The listing builds one solid part. Answer for the finished solid, in the listing's coordinates (mm). A direction names the side the tool comes from. Give positions to 0.01 mm unless a question says otherwise; leave off trailing zeros. Write each loop counter-clockwise with the first axis right and the second up, starting at its lowest first coordinate (ties: lowest second). Pieces come first, ordered by that corner, then holes. Notation, with made-up numbers: (-36.75, 71) - (-13.75, 71) arc R30 cw to (-13.75, 96) - close; hole circle Ø5 at (49.25, 31). An arc over 180 degrees is marked (long way). Return JSON: item names as keys, results as strings.
from build123d import *

# Parameters (mm, degrees)
F1_DEPTH = 19.05
F2_R     = 2.5
F3_DEPTH = 22
F5_DEPTH = 25
F7_DEPTH = 5
F8_R     = 1.8568549072
F9_DEPTH = 5


with BuildPart() as f1:
    # F0 (on Right) → F1 (new body)
    with BuildSketch(Plane.YZ):
        with BuildLine():
            Line((25, 0), (25, 1.9))
            Line((25, 1.9), (-25, 1.9))
            ThreePointArc((-25, 1.9), (-27.3925963531, 3.5206705817), (-26.8228433758, 6.3537734721))
            Line((-26.8228433758, 6.3537734721), (-9.338179633, 23.8384372149))
            Line((-9.338179633, 23.8384372149), (-10.6816825172, 25.1819400992))
            Line((-10.6816825172, 25.1819400992), (-28.3593520469, 7.5042705695))
            ThreePointArc((-28.3593520469, 7.5042705695), (-29.2640479302, 2.5952189514), (-25.0000004369, 0))
            Line((-25.0000004369, 0), (25, 0))
        make_face()
    extrude(amount=F1_DEPTH)

    # F2 (on face) → F3 (cut)
    with BuildSketch(Plane(origin=(0, 0, 0), x_dir=(1, 0, 0), z_dir=(0, 0, -1))):
        with BuildLine():
            Line((7.025, -5.5), (7.025, -20.5))
            ThreePointArc((7.025, -20.5), (9.525, -23), (12.025, -20.5))
            Line((12.025, -20.5), (12.025, -5.5))
            ThreePointArc((12.025, -5.5), (9.525, -3), (7.025, -5.5))
        make_face()
        with Locations((9.525, 7)):
            Circle(F2_R)
    extrude(amount=-F3_DEPTH, mode=Mode.SUBTRACT)

    # F4 (on face) → F5 (cut)
    with BuildSketch(Plane(origin=(0, 0, 0), x_dir=(1, 0, 0), z_dir=(0, 0, -1))):
        with BuildLine():
            ThreePointArc((2.0190405194, -25), (0.8550772375, -24.1079124506), (0, -22.9164958))
            Line((0, -22.9164958), (0, -25))
            Line((0, -25), (2.0190405194, -25))
        make_face()
        with BuildLine():
            ThreePointArc((19.05, -22.9164958), (18.1949227625, -24.1079124506), (17.0309594806, -25))
            Line((17.0309594806, -25), (19.05, -25))
            Line((19.05, -25), (19.05, -22.9164958))
        make_face()
    extrude(amount=-F5_DEPTH, mode=Mode.SUBTRACT)

    # F6 (on face) → F7 (cut)
    with BuildSketch(Plane(origin=(0, -17.9318113082, 17.9318113082), x_dir=(1, 0, 0), z_dir=(0, -0.7071067812, 0.7071067812))):
        with BuildLine():
            ThreePointArc((0, 7.3159923777), (0.8932364996, 9.0155780009), (2.3611190263, 10.2532304652))
            Line((2.3611190263, 10.2532304652), (0, 10.2532304652))
            Line((0, 10.2532304652), (0, 7.3159923777))
        make_face()
        with BuildLine():
            Line((19.05, 10.2532304652), (16.6888809737, 10.2532304652))
            ThreePointArc((16.6888809737, 10.2532304652), (18.1567635004, 9.0155780009), (19.05, 7.3159923777))
            Line((19.05, 7.3159923777), (19.05, 10.2532304652))
        make_face()
    extrude(amount=-F7_DEPTH, mode=Mode.SUBTRACT)

    # F8 (on face) → F9 (cut)
    with BuildSketch(Plane(origin=(0, -17.9318113082, 17.9318113082), x_dir=(1, 0, 0), z_dir=(0, -0.7071067812, 0.7071067812))):
        with Locations((4.5, 2.7532304652)):
            Circle(F8_R)
        with Locations((14.55, 2.7532304652)):
            Circle(F8_R)
    extrude(amount=-F9_DEPTH, mode=Mode.SUBTRACT)


solid = f1.part
Item 1: A cutting plane is placed at A-A on y = -7. Determine the outline of the cut face in (x, z) (3 decimals), then the cut area to 3 significant figures.
Answer below:
{"outline": "(0, 0) - (7.025, 0) - (7.025, 1.9) - (0, 1.9) - close; (12.025, 0) - (19.05, 0) - (19.05, 1.9) - (12.025, 1.9) - close", "area": "26.7 mm²"}
Item 2: Consider L1, parallel to X at y = -7, z = 0.7 (3 decimals); L2, parallel to Z at x = 13.5, y = 11; L3, parallel to Z at x = 16, y = -10. Determine where each line is inside the solid, lowest interval first.
Answer below:
{"L1": "x = 0 to 7.025, 12.025 to 19.05", "L2": "z = 0 to 1.9", "L3": "z = 0 to 1.9, 23.18 to 24.5"}
Item 3: A cutting plane is placed at D-D on y = 0. Determine the outline of the cut face in (x, z), then the cut area to 3 significant figures.
Answer below:
{"outline": "(0, 0) - (19.05, 0) - (19.05, 1.9) - (0, 1.9) - close", "area": "36.2 mm²"}
Item 4: Flat-ended cylindrical pins translate along their axes: P1, Ø6, axis at x = 16, y = -18.5, coming from the +Z side; P2, Ø5.5, axis at x = 7.5, y = -6.5, coming from the -Z side; P3, Ø2, axis at x = 6.5, z = 15, coming from the -Y side. Find the tip coordinate at first contact, or state that the pin passes through.
Answer below:
{"P1": "stops at z = 20.35", "P2": "stops at z = 0", "P3": "stops at y = -21.86"}
Item 5: A cutting plane is placed at B-B on x = 5.25. Determine the outline of the cut face in (y, z).
Answer below:
{"outline": "(-28.36, 7.5) arc R4.4 ccw to (-25, 0) - (25, 0) - (25, 1.9) - (-25, 1.9) arc R2.61 cw to (-26.82, 6.35) - (-15.84, 17.33) - (-17.19, 18.68) - close; (-14.78, 21.08) - (-13.44, 19.74) - (-9.34, 23.84) - (-10.68, 25.18) - close"}
Item 6: For faces 1 (the face through (9, 0, 1.9)), 2 (the face through (9.6, 3, 0.9)), 3 (the face through (16.32, -14.93, 19.61)), determine the directions among +Z, -Z, +X, -X, +Y, -Y from which every point of the face is accessible in a straight line to the end or side of a thin tool.
Answer below:
{"face 1": "+X, -X, +Y", "face 2": "+Z, -Z", "face 3": "none"}
Item 7: The mould has two halves that part along Z. Classify faces 4 (the face through (9.392, -19.397, 16.467)), 5 (the face through (19.05, -9, 1)), 6 (the face through (9.392, -18.203, 14.974)), 7 (the face through (9.392, -29.294, 2.663)): +Z half, -Z half, draft (parallel to the pull), parting line (faces both ways), or undercut.
Answer below:
{"face 4": "+Z half", "face 5": "draft", "face 6": "undercut", "face 7": "parting line"}
Item 8: A cutting plane is placed at C-C on y = -26. Determine the outline of the cut face in (x, z).
Answer below:
{"outline": "(0, 0.06) - (19.05, 0.06) - (19.05, 2.11) - (0, 2.11) - close; (0, 7.18) - (19.05, 7.18) - (19.05, 9.86) - (0, 9.86) - close"}
